```python
from build123d import *

# Parameters (mm, degrees)
ESQUISSE1_R             = 70
BOSS_EXTRU_1_DEPTH      = 150
ENL_V_MAT_EXTRU_1_DEPTH = 150
ENL_V_MAT_EXTRU_2_DEPTH = 180.008379692
ESQUISSE4_R             = 2.3
ENL_V_MAT_EXTRU_3_DEPTH = 20
ENL_V_MAT_EXTRU_4_DEPTH = 125
CHANFREIN1_SIZE         = 3
ESQUISSE6_R             = 8.5
ENL_V_MAT_EXTRU_5_DEPTH = 50


with BuildPart() as part:
    # Esquisse1 → Boss.-Extru.1 (new body)
    with BuildSketch(Plane(origin=(0, 0, 0), x_dir=(1, 0, 0), z_dir=(0, 1, 0))):
        with Locations(Location((0, 0, 0), (0, 0, 270))):
            Circle(ESQUISSE1_R)
    extrude(amount=-BOSS_EXTRU_1_DEPTH)

    # Esquisse2 → Enlèv. mat.-Extru.1 (cut)
    with BuildSketch(Plane(origin=(0, 0, 0), x_dir=(1, 0, 0), z_dir=(0, 1, 0))):
        with BuildLine():
            Line((-16, 68.14690015), (-16, 62.94690015))
            Line((-16, 62.94690015), (-8, 62.94690015))
            Line((-8, 62.94690015), (-8, 47.74690015))
            Line((-8, 47.74690015), (-12.8, 47.74690015))
            Line((-12.8, 47.74690015), (-12.8, 57.44690015))
            Line((-12.8, 57.44690015), (-16, 57.44690015))
            Line((-16, 57.44690015), (-16, -57.74690015))
            Line((-16, -57.74690015), (-12.8, -57.74690015))
            Line((-12.8, -57.74690015), (-12.8, -48.04690015))
            Line((-12.8, -48.04690015), (-8, -48.04690015))
            Line((-8, -48.04690015), (-8, -62.94690015))
            Line((-8, -62.94690015), (-16, -62.94690015))
            Line((-16, -62.94690015), (-16, -68.14690015))
            ThreePointArc((-16, -68.14690015), (70, 0), (-16, 68.14690015))
        make_face()
    extrude(amount=-ENL_V_MAT_EXTRU_1_DEPTH, mode=Mode.SUBTRACT)

    # Esquisse3 → Enlèv. mat.-Extru.2 (cut, through all)
    with BuildSketch(Plane(origin=(0, 0, 0), x_dir=(1, 0, 0), z_dir=(0, 1, 0))):
        Polygon((-27, 353.626649736), (-27, 64.58327957), (-27, 59.18327957), (-19.6, 59.18327957), (-19.6, 43.88327957), (-23, 43.88327957), (-23, 53.88327957), (-27, 53.88327957), (-27, -53.88327957), (-23, -53.88327957), (-23, -43.88327957), (-19.6, -43.88327957), (-19.6, -59.18327957), (-27, -59.18327957), (-27, -64.58327957), (-27, -353.626649736), (551.086740331, -353.626649736), (551.086740331, 353.626649736), align=None)
    extrude(amount=-ENL_V_MAT_EXTRU_2_DEPTH, mode=Mode.SUBTRACT)

    # Esquisse4 → Enlèv. mat.-Extru.3 (cut)
    with BuildSketch(Plane(origin=(-27, 0, 0), x_dir=(0, 0, -1), z_dir=(1, 0, 0))):
        with Locations((-11, -20)):
            Circle(ESQUISSE4_R)
        with Locations((11, -20)):
            Circle(ESQUISSE4_R)
    extrude(amount=-ENL_V_MAT_EXTRU_3_DEPTH, mode=Mode.SUBTRACT)

    # Esquisse5 → Enlèv. mat.-Extru.4 (cut)
    with BuildSketch(Plane.XZ.offset(150)):
        with BuildLine():
            Line((-27, 53.88327957), (-27, -53.88327957))
            Line((-27, -53.88327957), (-30, -53.88327957))
            ThreePointArc((-30, -53.88327957), (-67.584422787, 0), (-30, 53.88327957))
            Line((-30, 53.88327957), (-27, 53.88327957))
        make_face()
    extrude(amount=-ENL_V_MAT_EXTRU_4_DEPTH, mode=Mode.SUBTRACT)

    # Chanfrein1
    chanfrein1_edges = [part.edges().sort_by_distance(p)[0] for p in [
        (-70, 0, 0),
    ]]
    chamfer(chanfrein1_edges, length=CHANFREIN1_SIZE)

    # Esquisse6 → Enlèv. mat.-Extru.5 (cut)
    with BuildSketch(Plane(origin=(-27, 0, 0), x_dir=(0, 0, -1), z_dir=(1, 0, 0))):
        with Locations((-18.88327957, -12)):
            Circle(ESQUISSE6_R)
        with Locations((18.88327957, -12)):
            Circle(ESQUISSE6_R)
        with Locations((-0.00327957, -12)):
            Circle(ESQUISSE6_R)
    extrude(amount=-ENL_V_MAT_EXTRU_5_DEPTH, mode=Mode.SUBTRACT)


solid = part.part
```
The listing builds one solid part. Answer for the finished solid, in the listing's coordinates (mm). A direction names the side the tool comes from. Round coordinates to 2 decimals unless told otherwise and drop trailing zeros. Write each loop counter-clockwise with the first axis right and the second up, starting at its lowest first coordinate (ties: lowest second). Pieces come first, ordered by that corner, then holes. Notation, with made-up numbers: (-1, 63.5) -> (35, 63.5) arc R26 ccw to (35, 94.5) -> close; hole circle Ø1 at (77, 13.25). An arc over 180 degrees is marked (long way). Use CSV: the item, a comma, the result in double quotes. Start each with the question number.
(1) Each of these flat-tipped pins is pushed along its axis until it touches: pin 1 (1.7 mm diameter, centred on x = -22, y = -61.5, fed in from -Z); pin 2 (4 mm diameter, centred on y = -20, z = 11, fed in from -X); pin 3 (8 mm diameter, centred on y = -108.5, z = 46.5, fed in from -X). Where does it stop, or does it pass through?
(2) Consider L1, parallel to Z at x = -49.5, y = -12; L2, parallel to Z at x = -24, y = -20; L3, parallel to Z at x = -43.5, y = -12. Determine where each line is inside the solid, lowest interval first. Write a range as from..to.
(3) Section A-A on y = -12 is taken. Give the vertices of the cut face in (x, z), then the cut area to 3 significant figures.
(4) The mould has two halves that part along Y. Classify faces 6 (the face through (-27, -74, 62)), 7 (the face through (-47.817, -9.447, 10.776)), 8 (the face through (-42, -25, 1)): released by +Y, released by -Y, zero draft, split by the parting line, or undercut.
(5) Section C-C on x = -34 is taken. Count the separate pieces of the cut face and the enclosed holes in it, then the cut area to 3 significant figures.
(6) Which of the six approach directions +Z, -Z, +X, -X, +Y, -Y give full straight-line access (tool end or side, diameter ignored) to faces 1 (the face through (-27, -21, -1)), 2 (the face through (-67.576, -88.375, -0.979)), 3 (the face through (-23, -74, -59.183)), 4 (the face through (-47, -20, 11)), 5 (the face through (-23, -74, 59.183))?
(7) Section B-B on y = -113 is taken. Give the vertices of the cut face in (x, z), then the cut area to 3 significant figures.
A:
1,pin 1,"stops at z = -59.18"
1,pin 2,"stops at x = -69.42"
1,pin 3,"stops at x = -55.62"
2,L1,"z = -49.49..-27.38, -10.38..-8.5, 8.5..10.38, 27.38..49.49"
2,L2,"z = -59.18..-53.88, 53.88..59.18"
2,L3,"z = -54.84..-27.38, -10.38..-8.5, 8.5..10.38, 27.38..54.84"
3,outline,"(-69.48, -8.5) arc R70 ccw to (-69.23, -10.38) -> (-27, -10.38) -> (-27, -8.5) -> close; (-69.48, 8.5) -> (-27, 8.5) -> (-27, 10.38) -> (-69.23, 10.38) arc R70 ccw to start; (-64.42, -27.38) arc R70 ccw to (-27, -64.58) -> (-27, -59.18) -> (-19.6, -59.18) -> (-19.6, -43.88) -> (-23, -43.88) -> (-23, -53.88) -> (-27, -53.88) -> (-27, -27.38) -> close; (-64.42, 27.38) -> (-27, 27.38) -> (-27, 53.88) -> (-23, 53.88) -> (-23, 43.88) -> (-19.6, 43.88) -> (-19.6, 59.18) -> (-27, 59.18) -> (-27, 64.58) arc R70 ccw to start"
3,area,"2,060 mm²"
4,face 6,"zero draft"
4,face 7,"undercut"
4,face 8,"released by -Y"
5,separate pieces,"1"
5,enclosed holes,"5"
5,area,"4,570 mm²"
6,face 1,"+Y, -Y"
6,face 2,"-Y"
6,face 3,"-Z, +X, +Y, -Y"
6,face 4,"+X"
6,face 5,"+Z, +X, +Y, -Y"
7,outline,"(-30, -53.88) arc R57.42 cw to (-30, 53.88) -> (-23, 53.88) -> (-23, 43.88) -> (-19.6, 43.88) -> (-19.6, 59.18) -> (-27, 59.18) -> (-27, 64.58) arc R70 ccw to (-27, -64.58) -> (-27, -59.18) -> (-19.6, -59.18) -> (-19.6, -43.88) -> (-23, -43.88) -> (-23, -53.88) -> close"
7,area,"889 mm²"
